For this review, take the finished solid that the model builds, in its own axes (mm). A direction names the side the tool comes from. Coordinates: 2 decimals unless noted, no trailing zeros. Loops run counter-clockwise (first coordinate to the right, second up) from the corner with the lowest first, then second, coordinate; pieces in that order, holes last. Notation, with made-up numbers: (-22, 55) - (7, 55) arc R12 cw to (7, 77) - close; hole circle Ø4 at (-16.5, 29). An arc over 180 degrees is marked (long way). Answer as a JSON object with one key per item and string values. Group by question number.
Item 1: We need section A-A (y = 9). Give the boundary of the cut face in (x, z).
Item 2: Tool access review of faces 5 (the flat face through (0, 13, 2)), 6 (the flat face through (0, -16, 21)), 7 (the flat face through (-7, 12, 2)), 8 (the flat face through (0, 0, 0)), 9 (the flat face through (0, 14, 11)): name each direction out of +Z, -Z, +X, -X, +Y, -Y from which nothing blocks a thin tool from reaching the whole face with its end or side.
Item 3: We need section B-B (z = 5). Give the boundary of the cut face in (x, y), then the cut area to 3 significant figures.
Item 4: We need section D-D (z = 10.75). Give the boundary of the cut face in (x, y), then the cut area to 3 significant figures.
Item 5: Mouldability with a two-part tool opening along Y and no side actions: class faces 1 (the flat face through (7, 12, 2)), 2 (the flat face through (-6, 13.4, 4)), 3 (the flat face through (-7, 0, 12)), 4 (the flat face through (0, -14, 9)) as released by +Y, released by -Y, zero draft, split by the parting line, or undercut.
Item 6: Clearance check with flat-ended pins moving along their axes: pin 1 (4 mm diameter, centred on x = -2.5, y = -9, fed in from +Z); pin 2 (10 mm diameter, centred on x = 3, z = 6, fed in from +Y); pin 3 (0.8 mm diameter, centred on x = 0, z = 2.5, fed in from -Y). State where each tip first meets the part, or that it passes through.
Item 7: To check wall thickness, follow line 1 (X direction, y = 14.5, z = 20.35); line 2 (Y direction, x = 0, z = 19.85); line 3 (Z direction, x = -4, y = 13.5). State the ranges of each line that lie inside material, in increasing order.
from build123d import *

# Parameters (mm, degrees)
F0_W      = 17
F0_H      = 28
F0_W_2    = 14
F0_H_2    = 25
F1_DEPTH  = 23
F2_DEPTH  = 1.5
F3_W      = 17
F3_H      = 4
F4_DEPTH  = 4
F5_W      = 17
F5_H      = 4
F6_DEPTH  = 4
F5_W_2    = 12
F7_DEPTH  = 1.5
F8_SIZE   = 3.99999
F9_R      = 1.25
F10_DEPTH = 5
F11_R     = 4
F12_DEPTH = 25


# Not quite as in the source:
# - a fillet or chamfer is up to 0.001 mm smaller than in the source, because OpenCascade refuses the exact size


with BuildPart() as f1:
    # F0 (on Top) → F1 (new body)
    with BuildSketch(Plane.XY):
        Rectangle(F0_W, F0_H)
        Rectangle(F0_W_2, F0_H_2, mode=Mode.SUBTRACT)
    extrude(amount=F1_DEPTH)

    # F0 (on Top) → F2 (join)
    with BuildSketch(Plane.XY):
        Rectangle(F0_W_2, F0_H_2)
    extrude(amount=F2_DEPTH)

    # F3 (on face) → F4 (join)
    with BuildSketch(Plane.XZ.offset(14)):
        with Locations((0, 21)):
            Rectangle(F3_W, F3_H)
    extrude(amount=F4_DEPTH)

    # F5 (on face) → F6 (join)
    with BuildSketch(Plane(origin=(0, 14, 0), x_dir=(-1, 0, 0), z_dir=(0, 1, 0))):
        with Locations((0, 21)):
            Rectangle(F5_W, F5_H)
    extrude(amount=F6_DEPTH)

    # F5 (on face) → F7 (cut, through all)
    with BuildSketch(Plane(origin=(0, 14, 0), x_dir=(-1, 0, 0), z_dir=(0, 1, 0))):
        with Locations((0, 4)):
            Rectangle(F5_W_2, F5_H)
    extrude(amount=-F7_DEPTH, mode=Mode.SUBTRACT)

    # F8 (size 4 in the source; OpenCascade refuses exactly that, so slightly less here)
    f8_edges = [f1.edges().sort_by_distance(p)[0] for p in [
        (0, 18, 19),
        (0, -18, 19),
    ]]
    chamfer(f8_edges, length=F8_SIZE)

    # F9 (on face) → F10 (cut)
    with BuildSketch(Plane.XY.offset(23)):
        with Locations((0, 14.5)):
            Circle(F9_R)
        with Locations((0, -14.5)):
            Circle(F9_R)
    extrude(amount=-F10_DEPTH, mode=Mode.SUBTRACT)

    # F11 (on face) → F12 (cut)
    with BuildSketch(Plane(origin=(-8.5, 0, 0), x_dir=(0, -1, 0), z_dir=(-1, 0, 0))):
        with Locations((-9, 5)):
            Circle(F11_R)
    extrude(amount=-F12_DEPTH, mode=Mode.SUBTRACT)


solid = f1.part
Check sheet entries:
{
 "1": {"outline": "(-8.5, 0) - (8.5, 0) - (8.5, 1) - (-8.5, 1) - close; (-8.5, 9) - (-7, 9) - (-7, 23) - (-8.5, 23) - close; (7, 9) - (8.5, 9) - (8.5, 23) - (7, 23) - close"},
 "2": {"face 5": "+Y", "face 6": "-Z, +X, -X, -Y", "face 7": "+Z", "face 8": "-Z, +X, -X, +Y, -Y", "face 9": "-Z, +X, -X, +Y"},
 "3": {"outline": "(-8.5, -14) - (8.5, -14) - (8.5, 5) - (7, 5) - (7, -12.5) - (-7, -12.5) - (-7, 5) - (-8.5, 5) - close; (-8.5, 13) - (-6, 13) - (-6, 14) - (-8.5, 14) - close; (6, 13) - (8.5, 13) - (8.5, 14) - (6, 14) - close", "area": "83.0 mm2"},
 "4": {"outline": "(-8.5, -14) - (8.5, -14) - (8.5, 14) - (-8.5, 14) - close; hole (-7, -12.5) - (7, -12.5) - (7, 12.5) - (-7, 12.5) - close", "area": "126 mm2"},
 "5": {"face 1": "undercut", "face 2": "zero draft", "face 3": "undercut", "face 4": "released by -Y"},
 "6": {"pin 1": "stops at z = 1.5", "pin 2": "stops at y = 14", "pin 3": "stops at y = -14"},
 "7": {"line 1": "x = -8.5 to -1.25, 1.25 to 8.5", "line 2": "y = -13.25 to -12.5, 12.5 to 13.25", "line 3": "z = 0 to 2, 6 to 23"}
}
